Could you check a few things on this model? Use its own coordinates, in mm. A direction names the side the tool comes from. Give positions to 0.01 mm unless a question says otherwise; leave off trailing zeros. Write each loop counter-clockwise with the first axis right and the second up, starting at its lowest first coordinate (ties: lowest second). Pieces come first, ordered by that corner, then holes. Notation, with made-up numbers: (-22, 31) -> (11, 31) arc R18 cw to (11, 40) -> close; hole circle Ø5 at (23, -19.5). An arc over 180 degrees is marked (long way). One line per question, with ' | ' between items.
from build123d import *

# Parameters (mm, degrees)
CUT_EXTRUDE1_REACH      = 21.247
CUT_EXTRUDE1_END_RADIUS = 3.5
SKETCH5_R               = 2
SKETCH7_W               = 1
SKETCH7_H               = 12
CUT_EXTRUDE2_DEPTH      = 5.8


with BuildPart() as part:
    # Sweep1: sweep along a path in Sketch2
    with BuildLine(Plane(origin=(0, 0, 0), x_dir=(1, 0, 0), z_dir=(0, 1, 0))) as sweep1_path:
        CenterArc((0, 0), 5, 0, 360)
    # Sketch4 → Sweep1 (sweep)
    with BuildSketch(Plane(origin=(0, 0, 0), x_dir=(0, 0, -1), z_dir=(1, 0, 0))):
        Polygon((-2.4, 0), (-2.4, 3), (-0.75, 3), (-0.75, 5), (-2.5, 5), (-2.5, 13.8), (-6, 13.8), (-6, 8), (-5, 8), (-5, 0), align=None)
    sweep(path=sweep1_path.line)

    # Cut-Extrude1: up to this cylinder (the profile starts outside it)
    cut_extrude1_end = Plane(origin=(0, 10.9, 0), z_dir=(0, 1, 0)) * Cylinder(CUT_EXTRUDE1_END_RADIUS, 50.494, mode=Mode.PRIVATE)
    # Sketch5 → Cut-Extrude1 (cut, up to the surface)
    with BuildSketch(Plane(origin=(0, 13.8, 6), x_dir=(1, 0, 0), z_dir=(0, 0, 1)), mode=Mode.PRIVATE) as cut_extrude1_sk1:
        with Locations((0, -2.9)):
            Circle(SKETCH5_R)
    cut_extrude1_tool1 = extrude(cut_extrude1_sk1.sketch, amount=-CUT_EXTRUDE1_REACH, mode=Mode.PRIVATE) - cut_extrude1_end
    add(cut_extrude1_tool1.solids().sort_by_distance((0, 10.9, 6))[0], mode=Mode.SUBTRACT)

    # Sketch7 → Cut-Extrude2 (cut)
    with BuildSketch(Plane(origin=(0, 13.8, 0), x_dir=(1, 0, 0), z_dir=(0, 1, 0))):
        with Locations((-5.5, 0)):
            Rectangle(SKETCH7_W, SKETCH7_H)
        with Locations((5.5, 0)):
            Rectangle(SKETCH7_W, SKETCH7_H)
    extrude(amount=-CUT_EXTRUDE2_DEPTH, mode=Mode.SUBTRACT)


solid = part.part
Q1. If we mould it in two halves opening along Z, with no side actions, what happens to faces 4 (the cylindrical face through (0, 11, -6)), 5 (the cylindrical face through (4.77, 3.94, -1.5)), 6 (the cylindrical face through (-0.595, 4.014, 0.456)), 7 (the cylindrical face through (-2.398, 1.521, -0.106))? For each: +Z half, -Z half, draft (parallel to the pull), parting line (faces both ways), or undercut.
Answer below:
face 4: -Z half | face 5: parting line | face 6: undercut | face 7: undercut
Q2. Imagine slicing it at A-A on y = 10.9. Please give me the cut outline in (x, z).
Answer below:
outline: (-5, -3.32) arc R6 ccw to (5, -3.32) -> (5, 3.32) arc R6 ccw to (2, 5.66) -> (2, 2.87) arc R3.5 ccw to (-2, 2.87) -> (-2, 5.66) arc R6 ccw to (-5, 3.32) -> close; hole circle Ø5 at (0, 0)
Q3. Will these pins go through, and if not, where does the flat tip stop? pin 1 (5 mm diameter, centred on x = 3, y = 12, fed in from -Z); pin 2 (4 mm diameter, centred on x = 4, y = 7.5, fed in from +Z); pin 3 (1 mm diameter, centred on y = 4, z = 2, fed in from +X).
Answer below:
pin 1: stops at z = -5.98 | pin 2: stops at z = 5.63 | pin 3: stops at x = 4.77
Q4. If I drill on line 1 along Y through (x, z) = (0, 3.95); line 2 along Z through (x, y) = (0, 4.65); line 3 along Z through (x, y) = (0, 1.05), over which ranges is the centre line in solid material (lowest first)?
Answer below:
line 1: y = 0 to 8.9, 12.9 to 13.8 | line 2: z = -5 to -0.75, 0.75 to 5 | line 3: z = -5 to -2.4, 2.4 to 5
Q5. On a 3-axis mill with a long thin cutter (end or side, diameter ignored), from which of +Z, -Z, +X, -X, +Y, -Y can I reach the whole of each face in a straight line? I mean faces 1 (the cylindrical face through (2.385, 9.462, -0.751)), 2 (the flat face through (-5, 11, 0)), 3 (the cylindrical face through (1.847, 10.134, 4.458)). Say none if no direction works.
Answer below:
face 1: +Y | face 2: +Z, -Z, -X, +Y, -Y | face 3: +Z
Q6. Imagine slicing it at B-B on y = 8.25. Please give me the cut outline in (x, z).
Answer below:
outline: (-5, -3.32) arc R6 ccw to (5, -3.32) -> (5, 3.32) arc R6 ccw to (-5, 3.32) -> close; hole circle Ø5 at (0, 0)
